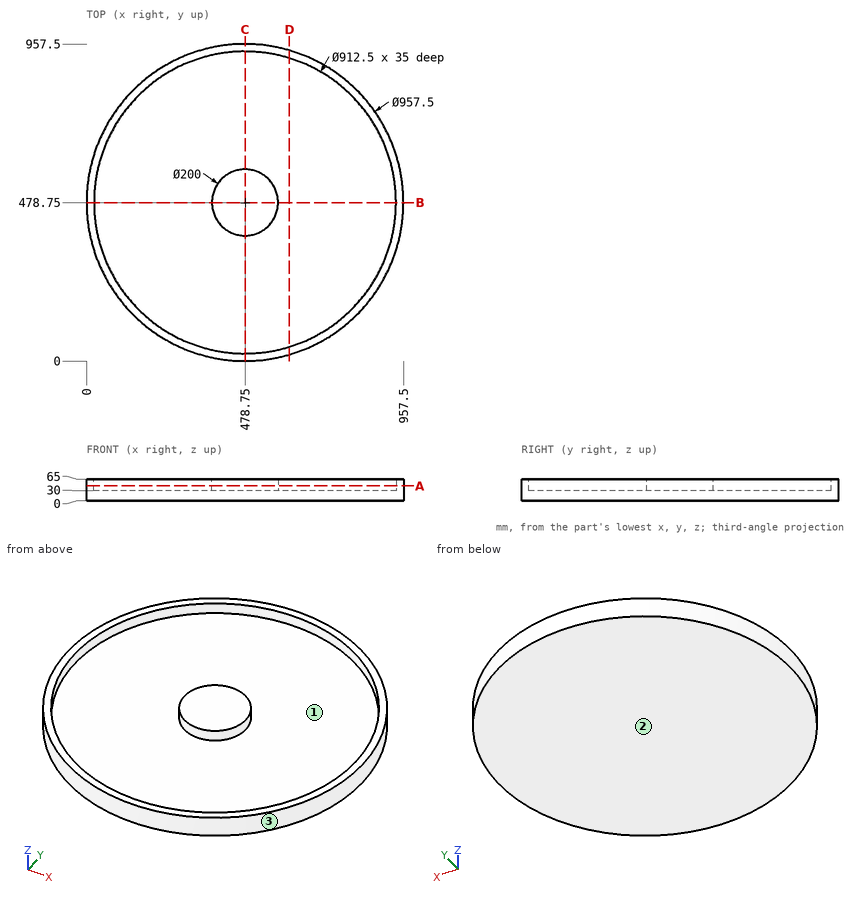
The drawing under review shows one solid part. Ordinate dimensions are in mm from its lowest x, y, z. Round coordinates to 2 decimals unless told otherwise and drop trailing zeros. Loops run counter-clockwise (first coordinate to the right, second up) from the corner with the lowest first, then second, coordinate; pieces in that order, holes last. Notation, with made-up numbers: (-6.75, 60) - (27.25, 60) arc R22 cw to (27.25, 70) - close; hole circle Ø7 at (56.5, -30.5). An arc over 180 degrees is marked (long way). One line per question, with ' | ' between items.
Q1. The part is to be moulded in two halves that separate along Y. For the marked faces 1, 2 and 3, say which applies: released by +Y, released by -Y, zero draft, split by the parting line, or undercut.
Taken from the geometry:
face 1: undercut | face 2: zero draft | face 3: split by the parting line
Q2. For line 1 along Y through (x, z) = (478.75, 43.5); line 2 along Z through (x, y) = (740.5, 200.5), list the stretches that pass through material, from the lowest coordinate up. Write a range as [from, to].
Taken from the geometry:
line 1: y = [0, 22.5], [378.75, 578.75], [935, 957.5] | line 2: z = [0, 30]
Q3. For pin 1 (2 mm diameter, centred on x = 114.5, z = 51.5, fed in from -Y); pin 2 (1 mm diameter, centred on x = 328.5, z = 26, fed in from +Y); pin 3 (4 mm diameter, centred on x = 578.5, y = 683.5, fed in from +Z), all flat-tipped, find the tip position at first contact; note any pin that passes through.
Taken from the geometry:
pin 1: stops at y = 166.9 | pin 2: stops at y = 933.48 | pin 3: stops at z = 30
Q4. Take a section at A-A (z = 44.5). Give the boundary of the cut face in (x, y).
Taken from the geometry:
outline: circle Ø957.5 at (478.75, 478.75); circle Ø200 at (478.75, 478.75); hole circle Ø912.5 at (478.75, 478.75)
Q5. Take a section at B-B (y = 478.75). Give the boundary of the cut face in (x, z), and give its area (3 significant figures).
Taken from the geometry:
outline: (0, 0) - (957.5, 0) - (957.5, 65) - (935, 65) - (935, 30) - (578.75, 30) - (578.75, 65) - (378.75, 65) - (378.75, 30) - (22.5, 30) - (22.5, 65) - (0, 65) - close | area: 37,300 mm²
Q6. Take a section at D-D (x = 612.5). Give the boundary of the cut face in (y, z), and give its area (3 significant figures).
Taken from the geometry:
outline: (19.06, 0) - (938.44, 0) - (938.44, 65) - (914.96, 65) - (914.96, 30) - (42.54, 30) - (42.54, 65) - (19.06, 65) - close | area: 29,200 mm²
